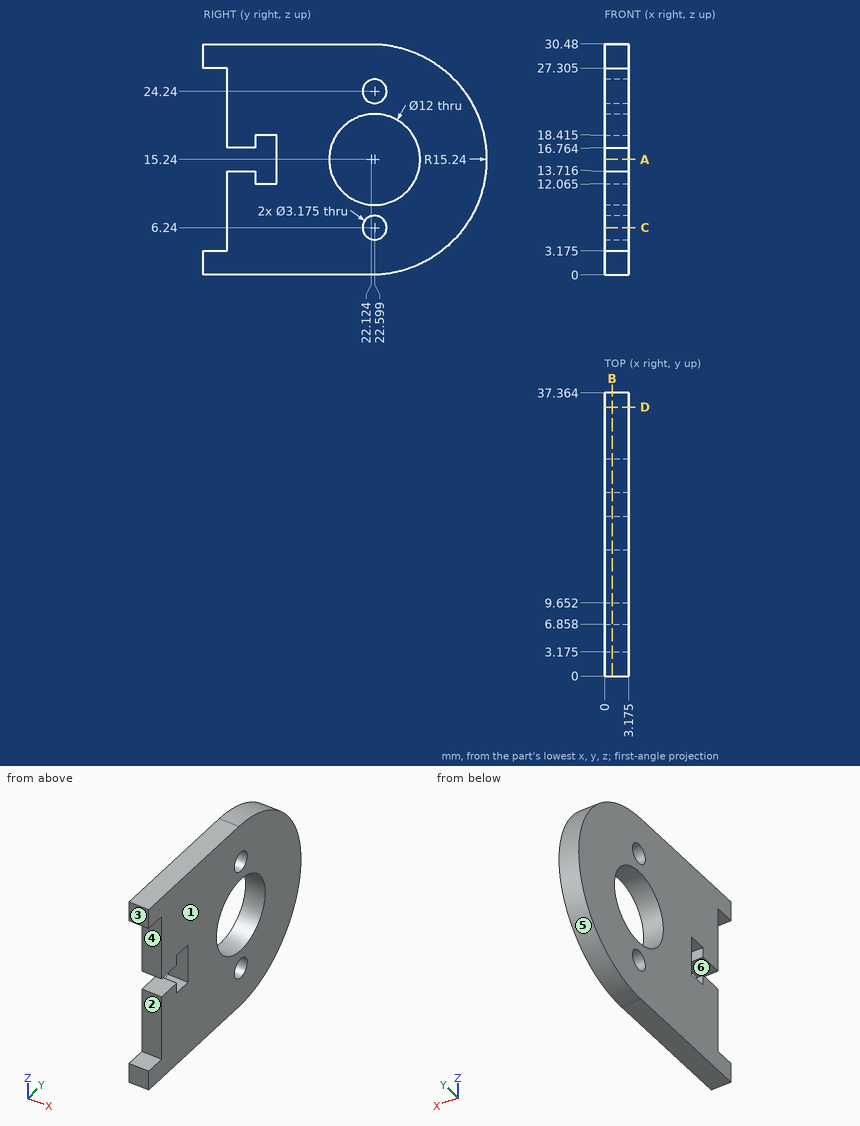
Input: dimensioned drawing with shaded views. Units: mm. Origin: part minimum x, y, z. A direction names the side the tool comes from. Give positions to 0.01 mm unless a question says otherwise; leave off trailing zeros. Write each loop counter-clockwise with the first axis right and the second up, starting at its lowest first coordinate (ties: lowest second). Pieces come first, ordered by that corner, then holes. Notation, with made-up numbers: M 37,77.5 L 71,77.5 A16 cw 71,96.5 Z; hole C -15.5,15 d6. An arc over 180 degrees is marked long. Write item = value, one per line. Start each with the question number.
1) Cut plane D-D on y = 35.5. Return the cut outline in (x, z) (3 decimals).
2) Cut plane B-B on x = 1. Return the cut outline in (y, z) (1 decimal), then the cut area to 3 significant figures.
3) Draft query along Z for the marked faces 3, 4, 5 and 6. Return one class per face: +Z half, -Z half, draft (parallel to the pull), parting line (faces both ways), or undercut.
4) Material intervals for line 1 along Z through (x, y) = (0.85, 3) (3 decimals); line 2 along Y through (x, z) = (2.5, 15.24); line 3 along Z through (x, y) = (1.05, 3.5), sorted ascending. Write a range as [from, to].
5) Cut plane C-C on z = 6.24. Return the cut outline in (x, y) (1 decimal).
6) First-contact query: pin 1 Ø0.8 at (x, z) = (1.5, 17.5) entering from +Y; pin 2 Ø1.8 at (x, z) = (2, 12.5) entering from +Y; pin 3 Ø1.9 at (y, z) = (22.6, 24.24) entering from +X; pin 4 Ø1 at (x, z) = (1.5, 16.5) entering from -Y (3 decimals). Flat tips, straight axial feed; report the tip coordinate or a pass-through.
7) Reachability of the marked faces 1 and 2 from +Z, -Z, +X, -X, +Y, -Y: full face, straight path, thin tool, end or side. Return the list, or none.
8) Cut plane A-A on z = 15.24. Return the cut outline in (x, y) (1 decimal).
Solved:
q1.outline = M 0,7.937 L 3.175,7.937 L 3.175,22.543 L 0,22.543 Z
q2.outline = M 0,0 L 22.1,0 A15.2 ccw 22.1,30.5 L 0,30.5 L 0,27.3 L 3.2,27.3 L 3.2,16.8 L 6.9,16.8 L 6.9,18.4 L 9.7,18.4 L 9.7,12.1 L 6.9,12.1 L 6.9,13.7 L 3.2,13.7 L 3.2,3.2 L 0,3.2 Z; hole C 22.6,15.2 d12; hole C 22.6,6.2 d3.2; hole C 22.6,24.2 d3.2
q2.area = 805 mm2
q3.face_3 = draft
q3.face_4 = undercut
q3.face_5 = parting line
q3.face_6 = undercut
q4.line_1 = [0, 3.175], [27.305, 30.48]
q4.line_2 = [9.65, 16.6], [28.6, 37.36]
q4.line_3 = [0, 13.72], [16.76, 30.48]
q5.outline = M 0,3.2 L 3.2,3.2 L 3.2,21 L 0,21 Z; M 0,24.2 L 3.2,24.2 L 3.2,34.4 L 0,34.4 Z
q6.pin_1 = 37.25
q6.pin_2 = 37.25
q6.pin_3 = through
q6.pin_4 = 3.175
q7.face_1 = +Z, -Z, +X, +Y, -Y
q7.face_2 = +X, -X, -Y
q8.outline = M 0,9.7 L 3.2,9.7 L 3.2,16.6 L 0,16.6 Z; M 0,28.6 L 3.2,28.6 L 3.2,37.4 L 0,37.4 Z
